Design review of the part shown in the three views and the two pictorial views. Dimensions are in mm from the part's minimum x, y and z. A direction names the side the tool comes from. Coordinates: 2 decimals unless noted, no trailing zeros. Loops run counter-clockwise (first coordinate to the right, second up) from the corner with the lowest first, then second, coordinate; pieces in that order, holes last. Notation, with made-up numbers: (74, 69) -> (94, 69) arc R21 ccw to (94, 91) -> close; hole circle Ø6 at (-13.5, -7.5). An arc over 180 degrees is marked (long way). Use CSV: the item, a comma, the result in double quotes.
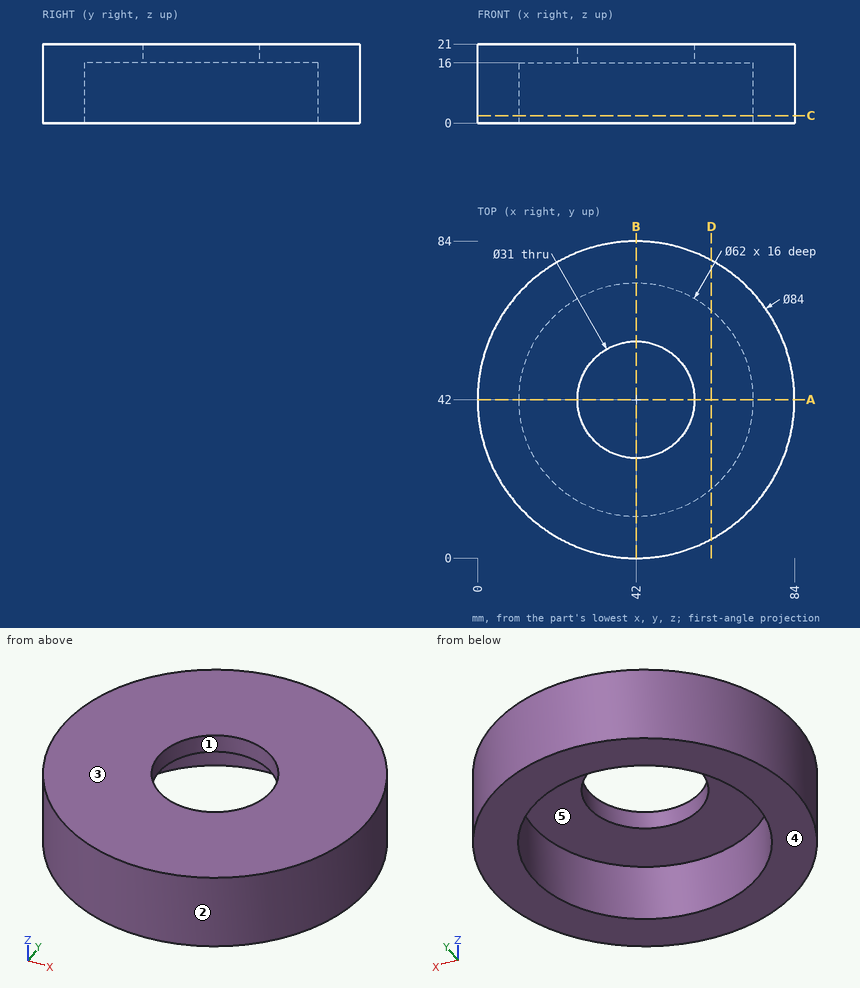
Item 1: Add section D-D (x = 62). Give the boundary of the cut face in (y, z).
Checked values:
outline,"(5.07, 0) -> (18.31, 0) -> (18.31, 16) -> (65.69, 16) -> (65.69, 0) -> (78.93, 0) -> (78.93, 21) -> (5.07, 21) -> close"
Item 2: To check wall thickness, follow line 1 along Y through (x, z) = (42, 3.5); line 2 along Z through (x, y) = (34, 63.5); line 3 along Y through (x, z) = (42, 18.95). State the ranges of each line that lie inside material, in increasing order.
Checked values:
line 1,"0 to 11, 73 to 84"
line 2,"16 to 21"
line 3,"0 to 26.5, 57.5 to 84"
Item 3: Clearance check with flat-ended pins moving along their axes: pin 1 (3 mm diameter, centred on x = 72.5, z = 13.5, fed in from -Y); pin 2 (12 mm diameter, centred on x = 45, y = 52, fed in from -Z); pin 3 (5 mm diameter, centred on y = 38, z = 12.5, fed in from +X). State where each tip first meets the part, or that it passes through.
Checked values:
pin 1,"y = 11.62"
pin 2,"z = 16"
pin 3,"x = 83.97"
Item 4: Add section A-A (y = 42). Give the boundary of the cut face in (x, z).
Checked values:
outline,"(0, 0) -> (11, 0) -> (11, 16) -> (26.5, 16) -> (26.5, 21) -> (0, 21) -> close; (57.5, 16) -> (73, 16) -> (73, 0) -> (84, 0) -> (84, 21) -> (57.5, 21) -> close"
Item 5: Add section C-C (z = 2). Give the boundary of the cut face in (x, y), then the cut area to 3 significant figures.
Checked values:
outline,"circle Ø84 at (42, 42); hole circle Ø62 at (42, 42)"
area,"2,520 mm^2"
Item 6: Machinability: for the marked faces 4 and 5, which of the approach directions +Z, -Z, +X, -X, +Y, -Y give a long, thin tool a straight path to every point of the face, cutting with its end or side? Answer none if there is none.
Checked values:
face 4,"-Z, +X, -X, +Y, -Y"
face 5,"-Z"
Item 7: Draft analysis for pull direction X (two halves, no side actions). For the marked faces 1, 2 and 3, state which applies: pulls with the +X half, pulls with the -X half, needs draft (parallel to the pull), parting line crosses it, or undercut.
Checked values:
face 1,"undercut"
face 2,"parting line crosses it"
face 3,"needs draft"
